from build123d import *

# Parameters (mm, degrees)
BOSS_EXTRUDE1_DEPTH = 6.35


with BuildPart() as part:
    # Model → Boss-Extrude1 (new body)
    with BuildSketch(Plane.XY):
        with BuildLine():
            Line((139.469217612, 83.486362243), (4.35423024, 165.635434247))
            ThreePointArc((4.35423024, 165.635434247), (3.5394e-05, 174.675549878), (6.482970516, 182.334156514))
            ThreePointArc((6.482970516, 182.334156514), (58.908007818, 222.053078132), (95.825996702, 276.486885341))
            ThreePointArc((95.825996702, 276.486885341), (123.003890417, 408.759091988), (116.719131272, 543.648218164))
            ThreePointArc((116.719131272, 543.648218164), (89.103473976, 723.73196509), (80.962507049, 905.738847083))
            ThreePointArc((80.962507049, 905.738847083), (74.958277304, 949.493417753), (54.91633926, 988.848645472))
            ThreePointArc((54.91633926, 988.848645472), (54.118865208, 993.201988834), (55.442796407, 997.425112023))
            ThreePointArc((55.442796407, 997.425112023), (58.582805567, 1000.544071106), (62.814738375, 1001.839566375))
            ThreePointArc((62.814738375, 1001.839566375), (106.978203286, 1002.158308411), (148.58698904, 1016.964461777))
            ThreePointArc((148.58698904, 1016.964461777), (313.920210211, 1093.500116289), (486.508708777, 1151.860981578))
            ThreePointArc((486.508708777, 1151.860981578), (587.939865291, 1195.825963048), (678.370898182, 1259.413913146))
            ThreePointArc((678.370898182, 1259.413913146), (696.610717819, 1275.98343537), (714.0803802, 1293.363049389))
            ThreePointArc((714.0803802, 1293.363049389), (745.41657129, 1351.190554942), (756.55215934, 1416.013204913))
            ThreePointArc((756.55215934, 1416.013204913), (758.517530867, 1423.598388709), (765.609904332, 1426.92944516))
            Line((765.609904332, 1426.92944516), (841.675709374, 1426.92944516))
            Line((841.675709374, 1426.92944516), (917.741514416, 1426.92944516))
            ThreePointArc((917.741514416, 1426.92944516), (924.83388788, 1423.598388709), (926.799259407, 1416.013204913))
            ThreePointArc((926.799259407, 1416.013204913), (937.934847458, 1351.190554942), (969.271038547, 1293.363049389))
            ThreePointArc((969.271038547, 1293.363049389), (986.740700928, 1275.98343537), (1004.980520565, 1259.413913146))
            ThreePointArc((1004.980520565, 1259.413913146), (1095.411553456, 1195.825963048), (1196.84270997, 1151.860981578))
            ThreePointArc((1196.84270997, 1151.860981578), (1369.431208537, 1093.500116289), (1534.76442971, 1016.964461776))
            ThreePointArc((1534.76442971, 1016.964461776), (1576.373215463, 1002.15830841), (1620.536680372, 1001.839566375))
            ThreePointArc((1620.536680372, 1001.839566375), (1624.76861318, 1000.544071106), (1627.90862234, 997.425112023))
            ThreePointArc((1627.90862234, 997.425112023), (1629.232553539, 993.201988834), (1628.435079487, 988.848645472))
            ThreePointArc((1628.435079487, 988.848645472), (1608.393141444, 949.493417753), (1602.388911699, 905.738847083))
            ThreePointArc((1602.388911699, 905.738847083), (1594.247944771, 723.73196509), (1566.632287475, 543.648218164))
            ThreePointArc((1566.632287475, 543.648218164), (1560.34752833, 408.759091988), (1587.525422045, 276.486885341))
            ThreePointArc((1587.525422045, 276.486885341), (1624.443410929, 222.053078132), (1676.868448231, 182.334156514))
            ThreePointArc((1676.868448231, 182.334156514), (1683.351383353, 174.675549878), (1678.997188507, 165.635434247))
            Line((1678.997188507, 165.635434247), (1543.882201136, 83.486362243))
            Line((1543.882201136, 83.486362243), (1408.767213764, 1.33729024))
            ThreePointArc((1408.767213764, 1.33729024), (1398.737467268, 1.632058994), (1394.921697237, 10.912285417))
            ThreePointArc((1394.921697237, 10.912285417), (1383.786109187, 75.734935389), (1352.449918097, 133.562440942))
            ThreePointArc((1352.449918097, 133.562440942), (1334.980255717, 150.942054961), (1316.740436079, 167.511577185))
            ThreePointArc((1316.740436079, 167.511577185), (1226.309403191, 231.099527281), (1124.878246681, 275.064508752))
            ThreePointArc((1124.878246681, 275.064508752), (1018.448935155, 308.599892952), (914.454996104, 349.060750407))
            ThreePointArc((914.454996104, 349.060750407), (878.82032779, 360.181940267), (841.675709373, 363.895129261))
            ThreePointArc((841.675709373, 363.895129261), (804.531090958, 360.181940267), (768.896422643, 349.060750407))
            ThreePointArc((768.896422643, 349.060750407), (664.902483594, 308.599892952), (558.47317207, 275.064508752))
            ThreePointArc((558.47317207, 275.064508752), (457.042015558, 231.099527282), (366.610982668, 167.511577185))
            ThreePointArc((366.610982668, 167.511577185), (348.371163031, 150.942054961), (330.90150065, 133.562440942))
            ThreePointArc((330.90150065, 133.562440942), (299.56530956, 75.734935389), (288.42972151, 10.912285417))
            ThreePointArc((288.42972151, 10.912285417), (284.613951479, 1.632058994), (274.584204983, 1.33729024))
            Line((274.584204983, 1.33729024), (139.469217612, 83.486362243))
        make_face()
        with BuildLine():
            Line((176.176913889, 204.976845914), (219.666503461, 276.506507813))
            ThreePointArc((219.666503461, 276.506507813), (249.41858659, 355.319849433), (248.604010602, 439.557998355))
            ThreePointArc((248.604010602, 439.557998355), (223.92684494, 569.757162888), (201.250512588, 700.319672443))
            ThreePointArc((201.250512588, 700.319672443), (200.544706813, 760.636081732), (212.373594943, 819.785424898))
            ThreePointArc((212.373594943, 819.785424898), (211.391671527, 852.848321028), (190.262486725, 878.297816581))
            Line((190.262486725, 878.297816581), (187.019990651, 880.269234028))
            ThreePointArc((187.019990651, 880.269234028), (176.385152977, 923.892911403), (220.008830352, 934.527749077))
            Line((220.008830352, 934.527749077), (223.251326425, 932.55633163))
            ThreePointArc((223.251326425, 932.55633163), (255.569588475, 925.510111894), (285.374887402, 939.854568323))
            ThreePointArc((285.374887402, 939.854568323), (332.444064978, 977.578034675), (386.318088828, 1004.710247))
            ThreePointArc((386.318088828, 1004.710247), (560.399041188, 1059.206662677), (735.592244912, 1110.013932483))
            ThreePointArc((735.592244912, 1110.013932483), (789.235659351, 1146.436483903), (809.925709373, 1207.886788985))
            Line((809.925709373, 1207.886788985), (809.925709373, 1238.443064765))
            ThreePointArc((809.925709373, 1238.443064765), (819.225069071, 1260.893705067), (841.675709374, 1270.193064765))
            ThreePointArc((841.675709374, 1270.193064765), (864.126349676, 1260.893705067), (873.425709374, 1238.443064765))
            Line((873.425709374, 1238.443064765), (873.425709374, 1207.886788985))
            ThreePointArc((873.425709374, 1207.886788985), (894.115759396, 1146.436483903), (947.759173836, 1110.013932483))
            ThreePointArc((947.759173836, 1110.013932483), (1122.952377559, 1059.206662677), (1297.03332992, 1004.710247))
            ThreePointArc((1297.03332992, 1004.710247), (1350.907353769, 977.578034675), (1397.976531346, 939.854568323))
            ThreePointArc((1397.976531346, 939.854568323), (1427.781830273, 925.510111903), (1460.100092322, 932.55633163))
            Line((1460.100092322, 932.55633163), (1463.342588395, 934.527749077))
            ThreePointArc((1463.342588395, 934.527749077), (1506.96626577, 923.892911403), (1496.331428096, 880.269234028))
            Line((1496.331428096, 880.269234028), (1493.088932022, 878.297816581))
            ThreePointArc((1493.088932022, 878.297816581), (1471.959747212, 852.848321031), (1470.977823804, 819.785424898))
            ThreePointArc((1470.977823804, 819.785424898), (1482.806711935, 760.636081732), (1482.100906159, 700.319672443))
            ThreePointArc((1482.100906159, 700.319672443), (1459.424573808, 569.757162888), (1434.747408146, 439.557998355))
            ThreePointArc((1434.747408146, 439.557998355), (1433.932832157, 355.319849433), (1463.684915286, 276.506507814))
            Line((1463.684915286, 276.506507814), (1507.174504858, 204.976845914))
            ThreePointArc((1507.174504858, 204.976845914), (1496.539667184, 161.353168539), (1452.915989809, 171.988006214))
            Line((1452.915989809, 171.988006214), (1409.426400237, 243.517668114))
            ThreePointArc((1409.426400237, 243.517668114), (1353.148046842, 306.20320239), (1277.986129436, 344.248115849))
            ThreePointArc((1277.986129436, 344.248115849), (1151.037755853, 382.25989552), (1024.687626725, 422.215243331))
            ThreePointArc((1024.687626725, 422.215243331), (957.191769225, 462.706773525), (911.118304628, 526.522842482))
            ThreePointArc((911.118304628, 526.522842482), (906.432646335, 531.976812223), (899.536415282, 534.012291743))
            Line((899.536415282, 534.012291743), (886.352318699, 534.012291743))
            ThreePointArc((886.352318699, 534.012291743), (877.372062578, 530.292547864), (873.652318699, 521.312291743))
            Line((873.652318699, 521.312291743), (873.652318699, 516.47003269))
            ThreePointArc((873.652318699, 516.47003269), (864.272697037, 493.939416342), (841.675709374, 484.72084139))
            ThreePointArc((841.675709374, 484.72084139), (819.078721711, 493.939416342), (809.699100048, 516.47003269))
            Line((809.699100048, 516.47003269), (809.699100048, 521.312291743))
            ThreePointArc((809.699100048, 521.312291743), (805.979356169, 530.292547864), (796.999100048, 534.012291743))
            Line((796.999100048, 534.012291743), (783.815003465, 534.012291743))
            ThreePointArc((783.815003465, 534.012291743), (776.918772408, 531.97681223), (772.23311412, 526.522842482))
            ThreePointArc((772.23311412, 526.522842482), (726.159649523, 462.706773525), (658.663792022, 422.215243331))
            ThreePointArc((658.663792022, 422.215243331), (532.313662894, 382.25989552), (405.365289309, 344.248115848))
            ThreePointArc((405.365289309, 344.248115848), (330.203371904, 306.203202389), (273.92501851, 243.517668114))
            Line((273.92501851, 243.517668114), (230.435428938, 171.988006214))
            ThreePointArc((230.435428938, 171.988006214), (186.811751564, 161.353168539), (176.176913889, 204.976845914))
        make_face(mode=Mode.SUBTRACT)
    extrude(amount=BOSS_EXTRUDE1_DEPTH)


solid = part.part
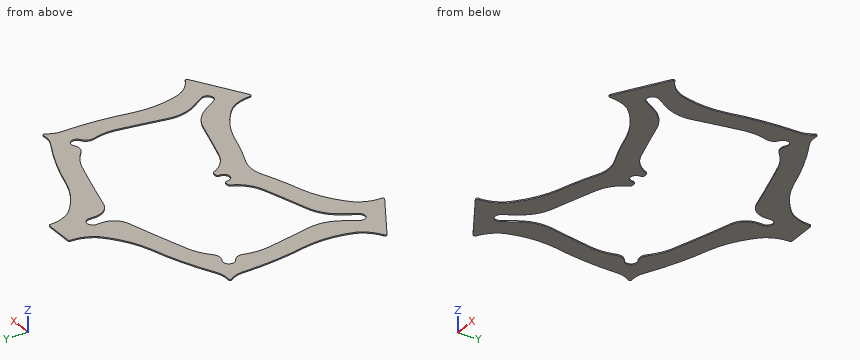
Could you check a few things on this model? Use its own coordinates, in mm. Round coordinates to 2 decimals unless told otherwise and drop trailing zeros. Order: outer loops, then holes, each group sorted by start corner. A loop starts at its lowest first (then second) coordinate and runs counter-clockwise, first axis right, second up.
Q1. I'm going to push flat-ended pins straight in: P1, Ø3, axis at y = 1224, z = 2, coming from the -X side; P2, Ø1.9, axis at y = 1224.5, z = 3, coming from the +X side. Where does each tip first touch, or does it pass through?
Geometry says:
P1: stops at x = 630.74
P2: stops at x = 1051.1
Q2. Imagine slicing it at C-C, the plane y = 1041.5. List the corners of the cut face in (x, z) for me, then the cut area to 3 significant figures.
Geometry says:
outline: (196.73, 0) - (502.41, 0) - (502.41, 6.35) - (196.73, 6.35) - close; (1180.94, 0) - (1486.62, 0) - (1486.62, 6.35) - (1180.94, 6.35) - close
area: 3,880 mm2
Q3. Imagine slicing it at A-A, the plane y = 312. List the corners of the cut face in (x, z) for me, then the cut area to 3 significant figures.
Geometry says:
outline: (106.54, 0) - (237.23, 0) - (237.23, 6.35) - (106.54, 6.35) - close; (338.11, 0) - (674.48, 0) - (674.48, 6.35) - (338.11, 6.35) - close; (1008.87, 0) - (1345.24, 0) - (1345.24, 6.35) - (1008.87, 6.35) - close; (1446.12, 0) - (1576.81, 0) - (1576.81, 6.35) - (1446.12, 6.35) - close
area: 5,930 mm2
Q4. Imagine slicing it at D-D, the plane y = 1332.5. List the corners of the cut face in (x, z) for me.
Geometry says:
outline: (737.88, 0) - (945.47, 0) - (945.47, 6.35) - (737.88, 6.35) - close
Q5. Imagine slicing it at B-B, the plane x = 515. List the corners of the cut face in (y, z) for me, then the cut area to 3 significant figures.
Geometry says:
outline: (259.21, 0) - (376.95, 0) - (376.95, 6.35) - (259.21, 6.35) - close; (1045.38, 0) - (1161.77, 0) - (1161.77, 6.35) - (1045.38, 6.35) - close
area: 1,490 mm2
Q6. Please list where these lines run through material, in increasing order: probe 1 along Y at (x, z) = (840.5, 4.5); probe 2 along Y at (x, z) = (997.5, 3.5); probe 3 along X at (y, z) = (858, 1.5).
Geometry says:
probe 1: y = 363.89 to 484.73, 1270.17 to 1426.93
probe 2: y = 316.12 to 434.15, 1096 to 1266.03
probe 3: x = 81.2 to 209.11, 1474.24 to 1602.15
